For this review, take the finished solid that the model builds, in its own axes (mm). Round coordinates to 2 decimals unless told otherwise and drop trailing zeros. Order: outer loops, then holes, each group sorted by start corner. A loop starts at its lowest first (then second) coordinate and runs counter-clockwise, first axis right, second up. Notation, with made-up numbers: M -18,-30.5 L 14,-30.5 A18 cw 14,0.5 Z; hole C -18.5,-35 d7. An arc over 180 degrees is marked long. Answer as a JSON object with one key per item and string values.
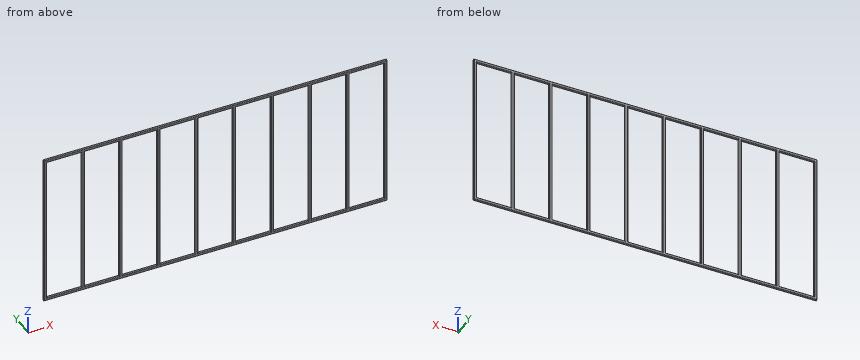
from build123d import *

# Parameters (mm, degrees)
F0_W     = 1360
F0_H     = 600
F0_W_2   = 140
F0_H_2   = 580
F1_DEPTH = 10
F2_R     = 2


with BuildPart() as f1:
    # F0 (on Front) → F1 (new body)
    with BuildSketch(Plane.XZ):
        with Locations((621.074081, 267.701469)):
            Rectangle(F0_W, F0_H)
        with Locations((21.074081, 267.701469)):
            Rectangle(F0_W_2, F0_H_2, mode=Mode.SUBTRACT)
        with Locations((171.074081, 267.701469)):
            Rectangle(F0_W_2, F0_H_2, mode=Mode.SUBTRACT)
        with Locations((321.074081, 267.701469)):
            Rectangle(F0_W_2, F0_H_2, mode=Mode.SUBTRACT)
        with Locations((471.074081, 267.701469)):
            Rectangle(F0_W_2, F0_H_2, mode=Mode.SUBTRACT)
        with Locations((621.074081, 267.701469)):
            Rectangle(F0_W_2, F0_H_2, mode=Mode.SUBTRACT)
        with Locations((771.074081, 267.701469)):
            Rectangle(F0_W_2, F0_H_2, mode=Mode.SUBTRACT)
        with Locations((921.074081, 267.701469)):
            Rectangle(F0_W_2, F0_H_2, mode=Mode.SUBTRACT)
        with Locations((1071.074081, 267.701469)):
            Rectangle(F0_W_2, F0_H_2, mode=Mode.SUBTRACT)
        with Locations((1221.074081, 267.701469)):
            Rectangle(F0_W_2, F0_H_2, mode=Mode.SUBTRACT)
    extrude(amount=F1_DEPTH)

    # F2
    f2_edges = [f1.edges().sort_by_distance(p)[0] for p in [
        (1221.074081, -10, -22.298531),
        (1151.074081, -10, 267.701469),
        (1071.074081, -10, -22.298531),
        (1141.074081, -10, 267.701469),
        (1221.074081, 0, -22.298531),
        (1151.074081, 0, 267.701469),
        (621.074081, -10, -32.298531),
        (1301.074081, -10, 267.701469),
        (1301.074081, 0, 267.701469),
        (1291.074081, -10, 267.701469),
        (621.074081, 0, -32.298531),
        (1291.074081, 0, 267.701469),
        (1141.074081, 0, 267.701469),
        (1071.074081, 0, -22.298531),
        (1001.074081, 0, 267.701469),
        (991.074081, 0, 267.701469),
        (991.074081, -10, 267.701469),
        (921.074081, 0, -22.298531),
        (841.074081, 0, 267.701469),
        (841.074081, -10, 267.701469),
        (771.074081, 0, -22.298531),
        (851.074081, 0, 267.701469),
        (701.074081, 0, 267.701469),
        (691.074081, 0, 267.701469),
        (691.074081, -10, 267.701469),
        (621.074081, 0, -22.298531),
        (551.074081, 0, 267.701469),
        (541.074081, 0, 267.701469),
        (541.074081, -10, 267.701469),
        (471.074081, 0, -22.298531),
        (401.074081, 0, 267.701469),
        (391.074081, 0, 267.701469),
        (321.074081, 0, -22.298531),
        (391.074081, -10, 267.701469),
        (251.074081, 0, 267.701469),
        (241.074081, 0, 267.701469),
        (241.074081, -10, 267.701469),
        (171.074081, 0, -22.298531),
        (101.074081, 0, 267.701469),
        (91.074081, 0, 267.701469),
        (91.074081, -10, 267.701469),
        (21.074081, 0, -22.298531),
        (-48.925919, 0, 267.701469),
        (-58.925919, 0, 267.701469),
        (-58.925919, -10, 267.701469),
        (21.074081, -10, 557.701469),
        (621.074081, 0, 567.701469),
        (171.074081, 0, 557.701469),
        (171.074081, -10, 557.701469),
        (471.074081, -10, 557.701469),
        (471.074081, 0, 557.701469),
        (321.074081, -10, 557.701469),
        (321.074081, 0, 557.701469),
        (771.074081, -10, 557.701469),
        (771.074081, 0, 557.701469),
        (621.074081, -10, 557.701469),
        (621.074081, 0, 557.701469),
        (1071.074081, -10, 557.701469),
        (1071.074081, 0, 557.701469),
        (921.074081, -10, 557.701469),
        (921.074081, 0, 557.701469),
        (1221.074081, -10, 557.701469),
        (1221.074081, 0, 557.701469),
        (1001.074081, -10, 267.701469),
        (851.074081, -10, 267.701469),
        (701.074081, -10, 267.701469),
        (551.074081, -10, 267.701469),
        (401.074081, -10, 267.701469),
        (251.074081, -10, 267.701469),
        (101.074081, -10, 267.701469),
        (-48.925919, -10, 267.701469),
        (621.074081, -10, 567.701469),
        (921.074081, -10, -22.298531),
        (771.074081, -10, -22.298531),
        (621.074081, -10, -22.298531),
        (471.074081, -10, -22.298531),
        (321.074081, -10, -22.298531),
        (171.074081, -10, -22.298531),
        (21.074081, -10, -22.298531),
        (21.074081, 0, 557.701469),
    ]]
    fillet(f2_edges, radius=F2_R)


solid = f1.part
1) Insertion check: P1, Ø1, axis at y = -1.5, z = 328.5, coming from the +X side. The pin has a flat end and moves straight along its axis. Give the tip position at first contact, or say it passes through.
Geometry check:
{"P1": "stops at x = 1301.07"}
2) Add section B-B on z = 100. State how many separate pieces and enclosed holes the cut face has, and give its area (3 significant figures).
Geometry check:
{"separate pieces": "10", "enclosed holes": "0", "area": "966 mm²"}
3) Add section A-A on x = 679. State the section outline as (y, z) points.
Geometry check:
{"outline": "M -10,-30.3 A2 ccw -8,-32.3 L -2,-32.3 A2 ccw 0,-30.3 L 0,-24.3 A2 ccw -2,-22.3 L -8,-22.3 A2 ccw -10,-24.3 Z; M -10,559.7 A2 ccw -8,557.7 L -2,557.7 A2 ccw 0,559.7 L 0,565.7 A2 ccw -2,567.7 L -8,567.7 A2 ccw -10,565.7 Z"}
4) For L1, parallel to Z at x = 681, y = -9; L2, parallel to Z at x = 466.5, y = -1.5; L3, parallel to Y at x = 393, z = -8, list the stretches that pass through material, from the lowest coordinate up.
Geometry check:
{"L1": "z = -32.03 to -22.57, 557.97 to 567.43", "L2": "z = -32.24 to -22.36, 557.76 to 567.64", "L3": "y = -10 to 0"}
